from build123d import *

# Parameters (mm, degrees)
SKETCH_3_R          = 8.24
EXTRUDE_5_DEPTH     = 2.18
SKETCH_7_R          = 4.01
EXTRUDE_6_DEPTH     = 1.36
SKETCH_8_R          = 2.42
EXTRUDE_7_DEPTH     = 4.28
SKETCH_9_R          = 5.6
CUT_EXTRUDE_3_DEPTH = 0.4
CUT_EXTRUDE_START   = -0.6
SKETCH_12_R         = 4.01
SKETCH_12_R_2       = 2.42
CUT_EXTRUDE_5_DEPTH = 0.6
SKETCH_13_OUTSIDE_W = 23.396
SKETCH_13_OUTSIDE_H = 23.396
SKETCH_13_OUTSIDE_R = 2.3
CUT_EXTRUDE_6_DEPTH = 4.88
SKETCH_14_R         = 2.3
CUT_EXTRUDE_7_DEPTH = 0.15


with BuildPart() as part:
    # 草图3 → 凸台-拉伸5 (new body)
    with BuildSketch(Plane(origin=(0, 0, 0), x_dir=(1, 0, 0), z_dir=(0, 1, 0))):
        with Locations(Location((0, 0, 0), (0, 0, 270))):
            Circle(SKETCH_3_R)
    extrude(amount=EXTRUDE_5_DEPTH)

    # 草图7 → 凸台-拉伸6 (add)
    with BuildSketch(Plane(origin=(0, 2.18, 0), x_dir=(1, 0, 0), z_dir=(0, 1, 0))):
        with Locations(Location((0, 0, 0), (0, 0, 270))):
            Circle(SKETCH_7_R)
    extrude(amount=EXTRUDE_6_DEPTH)

    # 草图8 → 凸台-拉伸7 (add)
    with BuildSketch(Plane(origin=(0, 3.54, 0), x_dir=(1, 0, 0), z_dir=(0, 1, 0))):
        with Locations(Location((0, 0, 0), (0, 0, 270))):
            Circle(SKETCH_8_R)
    extrude(amount=EXTRUDE_7_DEPTH)

    # 草图9 → 切除-拉伸3 (cut)
    with BuildSketch(Plane.XZ):
        with Locations(Location((0, 0, 0), (0, 0, 270))):
            Circle(SKETCH_9_R)
    extrude(amount=-CUT_EXTRUDE_3_DEPTH, mode=Mode.SUBTRACT)

    # 草图10 → 切除-旋转1 (revolve, cut)
    with BuildSketch(Plane.XY, mode=Mode.PRIVATE) as cut_revolve_1_sk:
        Polygon((5.6, 0.4), (6.6, 0), (5.6, 0), align=None)
    revolve(cut_revolve_1_sk.sketch.rotate(Axis((0, 7.82, 0), (0, -1, 0)), 90), axis=Axis((0, 7.82, 0), (0, -1, 0)), mode=Mode.SUBTRACT)

    # 草图11 → 切除-旋转2 (revolve, cut)
    with BuildSketch(Plane.XY, mode=Mode.PRIVATE) as cut_revolve_2_sk:
        Polygon((8.24, 0), (8.24, 1), (7.24, 0), align=None)
    revolve(cut_revolve_2_sk.sketch.rotate(Axis((0, 2.18, 0), (0, -1, 0)), 90), axis=Axis((0, 2.18, 0), (0, -1, 0)), mode=Mode.SUBTRACT)

    # 草图12 → 切除-拉伸5 (cut)
    with BuildSketch(Plane(origin=(0, 3.54, 0), x_dir=(1, 0, 0), z_dir=(0, 1, 0)).offset(CUT_EXTRUDE_START)):
        with Locations(Location((0, 0, 0), (0, 0, 270))):
            Circle(SKETCH_12_R)
        with Locations(Location((0, 0, 0), (0, 0, 270))):
            Circle(SKETCH_12_R_2, mode=Mode.SUBTRACT)
    extrude(amount=CUT_EXTRUDE_5_DEPTH, mode=Mode.SUBTRACT)

    # 草图13 outside → 切除-拉伸6 (cut)
    with BuildSketch(Plane(origin=(0, 7.82, 0), x_dir=(1, 0, 0), z_dir=(0, 1, 0))):
        Rectangle(SKETCH_13_OUTSIDE_W, SKETCH_13_OUTSIDE_H)
        with Locations(Location((0, 0, 0), (0, 0, 270))):
            Circle(SKETCH_13_OUTSIDE_R, mode=Mode.SUBTRACT)
    extrude(amount=-CUT_EXTRUDE_6_DEPTH, mode=Mode.SUBTRACT)

    # 草图14 → 切除-拉伸7 (cut)
    with BuildSketch(Plane(origin=(0, 7.82, 0), x_dir=(1, 0, 0), z_dir=(0, 1, 0))):
        with Locations(Location((0, 0, 0), (0, 0, 270))):
            Circle(SKETCH_14_R)
    extrude(amount=-CUT_EXTRUDE_7_DEPTH, mode=Mode.SUBTRACT)


solid = part.part
Geometry: final body of the model. Coordinates: model frame, mm. A direction names the side the tool comes from. Coordinates: 2 decimals unless noted, no trailing zeros. Loops run counter-clockwise (first coordinate to the right, second up) from the corner with the lowest first, then second, coordinate; pieces in that order, holes last. Notation, with made-up numbers: M 1.25,-20.5 L 48.25,-20.5 A12 cw 48.25,-8.5 Z; hole C 21.5,-11 d11. An arc over 180 degrees is marked long. One line per item, written item: value. Start each with the question number.
1) Cut plane D-D (y = 4). Return loops of the section in (x, z).
2) Reachability of faces 1 (the cylindrical face through (-8.044, 1.582, -1.786)), 2 (the flat face through (2, 2.18, 4)) from +Z, -Z, +X, -X, +Y, -Y: full face, straight path, thin tool, end or side. Return the list, or none.
3) Cut plane B-B (z = 0). Return loops of the section in (x, y), then the cut area to 3 significant figures.
4) Pin query (flat end, axial travel): P1, Ø1.5, axis at y = 1, z = 2, coming from the +X side; P2, Ø4, axis at x = -2.5, z = -3.5, coming from the -Y side; P3, Ø1, axis at x = -1.5, y = 2, coming from the +Z side. Return the tip coordinate at first contact, or that it passes through.
5) Draft query along X for faces 3 (the flat face through (0, 0.4, 0)), 4 (the cylindrical face through (0.691, 5.338, 2.194)), 5 (the flat face through (-2, 2.94, 2)). Return one class per face: released by +X, released by -X, zero draft, split by the parting line, or undercut.
6) Cut plane A-A (x = 0). Return loops of the section in (y, z), then the cut area to 3 significant figures.
7) Cut plane C-C (y = 2.5). Return loops of the section in (x, z).
8) Material intervals for L1, parallel to Y at x = -3.5, z = -6.25; L2, parallel to Y at x = 0.5, z = -1.75; L3, parallel to Z at x = 1, y = 4, sorted ascending. Write a range as from..to.
Evaluation:
1. outline: C 0,0 d4.6
2. face 1: +Y, -Y
2. face 2: +Y
3. outline: M -8.24,1 L -7.24,0 L -6.6,0 L -5.6,0.4 L 5.6,0.4 L 6.6,0 L 7.24,0 L 8.24,1 L 8.24,2.18 L 4.01,2.18 L 4.01,2.94 L 2.3,2.94 L 2.3,7.67 L -2.3,7.67 L -2.3,2.94 L -4.01,2.94 L -4.01,2.18 L -8.24,2.18 Z
3. area: 57.9 mm^2
4. P1: x = 8.14
4. P2: y = 0.12
4. P3: z = 8.18
5. face 3: undercut
5. face 4: split by the parting line
5. face 5: zero draft
6. outline: M 0,-7.24 L 1,-8.24 L 2.18,-8.24 L 2.18,-4.01 L 2.94,-4.01 L 2.94,-2.3 L 7.67,-2.3 L 7.67,2.3 L 2.94,2.3 L 2.94,4.01 L 2.18,4.01 L 2.18,8.24 L 1,8.24 L 0,7.24 L 0,6.6 L 0.4,5.6 L 0.4,-5.6 L 0,-6.6 Z
6. area: 57.9 mm^2
7. outline: C 0,0 d8.02
8. L1: 0..2.18
8. L2: 0.4..7.67
8. L3: -2.07..2.07
